The listing builds one solid part. Answer for the finished solid, in the listing's coordinates (mm). A direction names the side the tool comes from. Round coordinates to 2 decimals unless told otherwise and drop trailing zeros. Write each loop counter-clockwise with the first axis right and the second up, starting at its lowest first coordinate (ties: lowest second). Pieces come first, ordered by that corner, then holes. Notation, with made-up numbers: M -2,67 L 32,67 A25 cw 32,101 Z; hole C -5,86.5 d6. An arc over 180 degrees is marked long. Put each result on its own line as item: value. Start each with the question number.
```python
from build123d import *

# Parameters (mm, degrees)
BOSS_EXTRUDE2_DEPTH = 11
SKETCH5_R           = 15
BOSS_EXTRUDE4_DEPTH = 25
SKETCH6_R           = 10
CUT_EXTRUDE1_DEPTH  = 20
SKETCH7_R           = 7.5
CUT_EXTRUDE2_DEPTH  = 289.149419546
SKETCH8_W           = 40.868784051
SKETCH8_H           = 7.083722135
BOSS_EXTRUDE5_DEPTH = 15
SKETCH9_W           = 36
SKETCH9_H           = 18
CUT_EXTRUDE3_DEPTH  = 5


with BuildPart() as part:
    # Sketch3 → Boss-Extrude2 (new body)
    with BuildSketch(Plane(origin=(0, 0, 0), x_dir=(1, 0, 0), z_dir=(0, 1, 0))):
        with BuildLine():
            Line((-266.757890885, 20), (-196.757890885, 20))
            ThreePointArc((-196.757890885, 20), (-176.757890885, 0), (-196.757890885, -20))
            Line((-196.757890885, -20), (-266.757890885, -20))
            ThreePointArc((-266.757890885, -20), (-286.757890885, 0), (-266.757890885, 20))
        make_face()
    extrude(amount=BOSS_EXTRUDE2_DEPTH)

    # Sketch5 → Boss-Extrude4 (add)
    with BuildSketch(Plane(origin=(0, 11, 0), x_dir=(1, 0, 0), z_dir=(0, 1, 0))):
        with Locations(Location((-196.757890885, 0, 0), (0, 0, 90))):
            Circle(SKETCH5_R)
        with Locations(Location((-266.757890885, 0, 0), (0, 0, 90))):
            Circle(SKETCH5_R)
    extrude(amount=BOSS_EXTRUDE4_DEPTH)

    # Sketch6 → Cut-Extrude1 (cut)
    with BuildSketch(Plane(origin=(0, 36, 0), x_dir=(1, 0, 0), z_dir=(0, 1, 0))):
        with Locations(Location((-266.757890885, 0, 0), (0, 0, 270))):
            Circle(SKETCH6_R)
        with Locations(Location((-196.757890885, 0, 0), (0, 0, 270))):
            Circle(SKETCH6_R)
    extrude(amount=-CUT_EXTRUDE1_DEPTH, mode=Mode.SUBTRACT)

    # Sketch7 → Cut-Extrude2 (cut, through all)
    with BuildSketch(Plane(origin=(0, 16, 0), x_dir=(1, 0, 0), z_dir=(0, 1, 0))):
        with Locations(Location((-196.757890885, 0, 0), (0, 0, 270))):
            Circle(SKETCH7_R)
        with Locations(Location((-266.757890885, 0, 0), (0, 0, 270))):
            Circle(SKETCH7_R)
    extrude(amount=-CUT_EXTRUDE2_DEPTH, mode=Mode.SUBTRACT)

    # Sketch8 → Boss-Extrude5 (add)
    with BuildSketch(Plane(origin=(0, 11, 0), x_dir=(1, 0, 0), z_dir=(0, 1, 0))):
        with Locations((-231.757890885, -0.041861068)):
            Rectangle(SKETCH8_W, SKETCH8_H)
    extrude(amount=BOSS_EXTRUDE5_DEPTH)

    # Sketch9 → Cut-Extrude3 (cut)
    with BuildSketch(Plane.XZ):
        with Locations((-231.107838077, 0.023445498)):
            Rectangle(SKETCH9_W, SKETCH9_H)
    extrude(amount=-CUT_EXTRUDE3_DEPTH, mode=Mode.SUBTRACT)


solid = part.part
```
Item 1: Which of the six approach directions +Z, -Z, +X, -X, +Y, -Y give full straight-line access (tool end or side, diameter ignored) to faces 1 (the cylindrical face through (-188.33, 26.14, 5.38)), 2 (the flat face through (-232, 18, -3.5)), 3 (the flat face through (-249.108, 2, 0))?
Item 2: Consider line 1 along X through (y, z) = (27, 0); line 2 along X through (y, z) = (22, 0); line 3 along X through (y, z) = (6.25, 0). Determine where each line is inside the solid, lowest interval first. Write a range as [from, to].
Item 3: Section A-A (z = 0) is taken. Count the separate pieces of the cut face and the enclosed holes in it, and give its area (3 significant figures).
Item 4: Section B-B (y = 20) is taken. Give the vertices of the cut face in (x, z), and give its area (3 significant figures).
Item 5: Section D-D (x = -216.5) is taken. Give the vertices of the cut face in (y, z).
Item 6: Section C-C (x = -200) is taken. Give the vertices of the cut face in (y, z), and give its area (3 significant figures).
Item 7: Flat-ended cylindrical pins translate along their axes: pin 1 (3 mm diameter, centred on y = 19, z = 10.5, fed in from +X); pin 2 (2 mm diameter, centred on x = -228, y = 11.5, fed in from +Z); pin 3 (2 mm diameter, centred on y = 9.5, z = -12.5, fed in from +X); pin 4 (8 mm diameter, centred on x = -235, z = 15.5, fed in from +Y). Find the tip coordinate at first contact, or state that the pin passes through.
Item 8: Determine the mould class of faces 4 (the flat face through (-232, 18, 3.584)), 5 (the flat face through (-264, 36, -10)), 6 (the cylindrical face through (-281.63, 23.32, 1.95)) for opening direction X: released by +X, released by -X, zero draft, split by the parting line, or undercut.
Output values:
1. face 1: +Y
1. face 2: -Z, +Y
1. face 3: -Y
2. line 1: x = [-281.76, -276.76], [-256.76, -251.76], [-211.76, -206.76], [-186.76, -181.76]
2. line 2: x = [-281.76, -276.76], [-256.76, -206.76], [-186.76, -181.76]
2. line 3: x = [-286.76, -274.26], [-259.26, -204.26], [-189.26, -176.76]
3. separate pieces: 3
3. enclosed holes: 0
3. area: 1,850 mm^2
4. outline: M -252.19,3.58 A15 ccw long -252.17,-3.5 L -211.34,-3.5 A15 ccw long -211.32,3.58 Z; hole C -266.76,0 d20; hole C -196.76,0 d20
4. area: 1,070 mm^2
5. outline: M 0,-20 L 11,-20 L 11,-3.5 L 26,-3.5 L 26,3.58 L 11,3.58 L 11,20 L 0,20 L 0,9.02 L 5,9.02 L 5,-8.98 L 0,-8.98 Z
6. outline: M 0,-20 L 11,-20 L 11,-14.65 L 36,-14.65 L 36,-9.46 L 16,-9.46 L 16,-6.76 L 0,-6.76 Z; M 0,6.76 L 16,6.76 L 16,9.46 L 36,9.46 L 36,14.65 L 11,14.65 L 11,20 L 0,20 Z
6. area: 577 mm^2
7. pin 1: stops at x = -184.76
7. pin 2: stops at z = 20
7. pin 3: stops at x = -180.39
7. pin 4: stops at y = 11
8. face 4: undercut
8. face 5: zero draft
8. face 6: undercut
